Autodesk Inventor part; units mm, degrees
ref_plane "YZ Plane" through (0, 0, 0) normal (1, 0, 0) x (0, 1, 0)
ref_plane "XZ Plane" through (0, 0, 0) normal (0, 1, 0) x (-1, 0, 0)
ref_plane "XY Plane" through (0, 0, 0) normal (0, 0, 1) x (1, 0, 0)
sketch "Sketch1" plane through (0, 0, 0) normal (0, 1, 0) x (-1, 0, 0)
  circle A0 centre (0, 0) radius 10
  dimension "d0" = 20
extrude "Extrusion1" add sketch "Sketch1" along normal blind 1.8
sketch "Sketch3" plane through (0, 1.8, 0) normal (0, 1, 0) x (1, 0, 0)
  circle A0 centre (0, 0) radius 10
  circle A1 centre (0, 0) radius 3.5
  circle A2 centre (0, 0) radius 2.5
  dimension "d3" = 7
  dimension "d4" = 5
extrude "Extrusion2" add sketch "Sketch3" along normal blind 2.4 contours A1
sketch "Sketch4" plane through (0, 0, 0) normal (0, -1, 0) x (1, 0, 0)
  circle A0 centre (0, 0) radius 10
  line L0 (0, 0) -> (6.3, 0)
  circle A1 centre (6.3, 0) radius 1.5
  dimension "d7" = 6.3
  dimension "d8" = 3
extrude "Extrusion3" cut sketch "Sketch4" against normal blind 2.4 contours A1
sketch "Sketch5" plane through (0, 0, 0) normal (0, -1, 0) x (1, 0, 0)
  circle A0 centre (0, 0) radius 10
  line L0 (0, 0) -> (-6.3, 0)
  circle A1 centre (-6.3, 0) radius 1.5
  dimension "d11" = 6.3
  dimension "d12" = 3
extrude "Extrusion4" cut sketch "Sketch5" against normal blind 2 contours A1
properties part number "paka2_micro"
Here's how the part is built. I have some questions about the finished solid (model axes, mm). A direction names the side the tool comes from. Coordinates: 2 decimals unless noted, no trailing zeros. Write each loop counter-clockwise with the first axis right and the second up, starting at its lowest first coordinate (ties: lowest second). Pieces come first, ordered by that corner, then holes.
Item 1: I want a section at A-A on z = 0. Write out the boundary of the cut face in (x, y), and give its area (3 significant figures).
Item 2: I want a section at D-D on y = 2.3. Write out the boundary of the cut face in (x, z), and give its area (3 significant figures).
Item 3: Will these pins go through, and if not, where does the flat tip stop? pin 1 (1 mm diameter, centred on x = -4.5, z = 3.5, fed in from -Y); pin 2 (1.5 mm diameter, centred on x = 0, z = 0.5, fed in from +Y).
Item 4: If I drill on line 1 (X direction, y = 2.7, z = 0); line 2 (X direction, y = 0.2, z = -1); line 3 (Y direction, x = 0.25, z = 6), over which ranges is the centre line in solid material (lowest first)?
Item 5: I want a section at C-C on x = 0. Write out the boundary of the cut face in (y, z), and give its area (3 significant figures).
Item 6: I want a section at B-B on x = -5.25. Write out the boundary of the cut face in (y, z).
Item 7: On a 3-axis mill with a long thin cutter (end or side, diameter ignored), from which of +Z, -Z, +X, -X, +Y, -Y can I reach the whole of each face in a straight line? I mean faces 1 (the cylindrical face through (3.233, 2.983, -1.341)), 2 (the flat face through (0, 0, 0)). Say none if no direction works.
Item 8: If we mould it in two halves opening along Z, with no side actions, what happens to faces 3 (the cylindrical face through (-4.87, 0.89, 0.45)), 4 (the flat face through (-4, 1.8, 0)), 5 (the cylindrical face through (2.17, 0.89, 9.76))? For each: +Z half, -Z half, draft (parallel to the pull), parting line (faces both ways), or undercut.
Findings below:
1. outline: (-10, 0) - (-7.8, 0) - (-7.8, 1.8) - (-10, 1.8) - close; (-4.8, 0) - (4.8, 0) - (4.8, 1.8) - (3.5, 1.8) - (3.5, 4.2) - (2.5, 4.2) - (2.5, 1.8) - (-2.5, 1.8) - (-2.5, 4.2) - (-3.5, 4.2) - (-3.5, 1.8) - (-4.8, 1.8) - close; (7.8, 0) - (10, 0) - (10, 1.8) - (7.8, 1.8) - close
1. area: 30.0 mm2
2. outline: circle Ø7 at (0, 0); hole circle Ø5 at (0, 0)
2. area: 18.8 mm2
3. pin 1: stops at y = 0
3. pin 2: stops at y = 1.8
4. line 1: x = -3.5 to -2.5, 2.5 to 3.5
4. line 2: x = -9.95 to -7.42, -5.18 to 5.18, 7.42 to 9.95
4. line 3: y = 0 to 1.8
5. outline: (0, -10) - (1.8, -10) - (1.8, -3.5) - (4.2, -3.5) - (4.2, -2.5) - (1.8, -2.5) - (1.8, 2.5) - (4.2, 2.5) - (4.2, 3.5) - (1.8, 3.5) - (1.8, 10) - (0, 10) - close
5. area: 40.8 mm2
6. outline: (0, -8.51) - (1.8, -8.51) - (1.8, -1.07) - (0, -1.07) - close; (0, 1.07) - (1.8, 1.07) - (1.8, 8.51) - (0, 8.51) - close
7. face 1: +Y
7. face 2: +Z, -Z, +X, -X, -Y
8. face 3: undercut
8. face 4: draft
8. face 5: parting line
